Geometry check sheet. Reference: the model listing, model coordinates, mm. A direction names the side the tool comes from. Coordinates: 2 decimals unless noted, no trailing zeros. Loops run counter-clockwise (first coordinate to the right, second up) from the corner with the lowest first, then second, coordinate; pieces in that order, holes last. Notation, with made-up numbers: (65.5, 61.5) -> (108.5, 61.5) arc R20 ccw to (108.5, 77.5) -> close; hole circle Ø8 at (-30, 73.25). An arc over 180 degrees is marked (long way). Answer as a JSON object with one key per item and string values.
from build123d import *

# Parameters (mm, degrees)
SKETCH2_W               = 3.175
SKETCH2_H               = 42.221697185
SKETCH3_W               = 3.175
SKETCH3_H               = 3.175
CUT_EXTRUDE1_DEPTH      = 1.27
CUT_EXTRUDE2_DEPTH      = 41.54574875
CUT_EXTRUDE2_DEPTH_BACK = 41.54574875


with BuildPart() as part:
    # Sketch2 → Revolve1 (revolve)
    with BuildSketch(Plane.XY, mode=Mode.PRIVATE) as revolve1_sk:
        with Locations((22.889936685, 21.110848593)):
            Rectangle(SKETCH2_W, SKETCH2_H)
    revolve(revolve1_sk.sketch.rotate(Axis((0, 38.094197185, 0), (0, -1, 0)), 180), axis=Axis((0, 38.094197185, 0), (0, -1, 0)))

    # Sketch3 → Cut-Extrude1 (cut)
    with BuildSketch(Plane(origin=(0, 42.221697185, 0), x_dir=(1, 0, 0), z_dir=(0, 1, 0))):
        with Locations((0, 24.425903267)):
            Rectangle(SKETCH3_W, SKETCH3_H)
        with Locations((0, -24.425903267)):
            Rectangle(SKETCH3_W, SKETCH3_H)
    cut_extrude1 = extrude(amount=-CUT_EXTRUDE1_DEPTH, mode=Mode.SUBTRACT)

    # Mirror1: Cut-Extrude1 across plane
    add(cut_extrude1.mirror(Plane.ZX.offset(21.110848593)), mode=Mode.SUBTRACT)

    # Sketch4 → Cut-Extrude2 (cut, two sides: drawn at the far end of the back side and taken through both)
    with BuildSketch(Plane(origin=(0, 21.110848593, 0), x_dir=(1, 0, 0), z_dir=(0, 1, 0)).offset(-CUT_EXTRUDE2_DEPTH_BACK)):
        with BuildLine():
            Line((24.472510779, 0.491042627), (23.622, 0))
            Line((23.622, 0), (24.472510779, -0.491042627))
            ThreePointArc((24.472510779, -0.491042627), (24.477436685, 0), (24.472510779, 0.491042627))
        make_face()
        with BuildLine():
            Line((21.26790239, 1.21249192), (23.368, 0))
            Line((23.368, 0), (21.26790239, -1.21249192))
            ThreePointArc((21.26790239, -1.21249192), (21.302436685, 0), (21.26790239, 1.21249192))
        make_face()
    extrude(amount=CUT_EXTRUDE2_DEPTH + CUT_EXTRUDE2_DEPTH_BACK, mode=Mode.SUBTRACT)


solid = part.part
1. Section check C-C, the plane y = 26.5. Record the boundary of the cut face in (x, z).
Evaluation:
{"outline": "(23.62, 0) -> (24.47, 0.49) arc R24.48 ccw (long way) to (24.47, -0.49) -> close; hole (21.27, -1.21) -> (23.37, 0) -> (21.27, 1.21) arc R21.3 ccw (long way) to start"}
2. Mould release check, pull along X, two halves, no side actions. Record for faces 1 (the face through (0, 1, 22.838)), 2 (the face through (0, 42.222, 22)): released by +X, released by -X, zero draft, split by the parting line, or undercut.
Evaluation:
{"face 1": "undercut", "face 2": "zero draft"}
3. Section check D-D, the plane x = 0. Record the boundary of the cut face in (y, z), then the cut area to 3 significant figures.
Evaluation:
{"outline": "(0, -22.84) -> (1.27, -22.84) -> (1.27, -24.48) -> (40.95, -24.48) -> (40.95, -22.84) -> (42.22, -22.84) -> (42.22, -21.3) -> (0, -21.3) -> close; (0, 21.3) -> (42.22, 21.3) -> (42.22, 22.84) -> (40.95, 22.84) -> (40.95, 24.48) -> (1.27, 24.48) -> (1.27, 22.84) -> (0, 22.84) -> close", "area": "260 mm^2"}
4. Section check A-A, the plane x = -19.5. Record the boundary of the cut face in (y, z), then the cut area to 3 significant figures.
Evaluation:
{"outline": "(0, -14.8) -> (42.22, -14.8) -> (42.22, -8.58) -> (0, -8.58) -> close; (0, 8.58) -> (42.22, 8.58) -> (42.22, 14.8) -> (0, 14.8) -> close", "area": "525 mm^2"}
5. Depth check by flat-ended pin: P1, Ø5, axis at x = 19, y = 9.5, coming from the -Z side; P2, Ø1, axis at x = 7, y = 17.5, coming from the +Z side; P3, Ø0.5, axis at x = 0.5, z = 23.5, coming from the -Y side. Enter the tip coordinate at first touch or a pass-through.
Evaluation:
{"P1": "stops at z = -18.08", "P2": "stops at z = 23.6", "P3": "stops at y = 1.27"}
6. Section check B-B, the plane z = -20.5. Record the boundary of the cut face in (x, y), then the cut area to 3 significant figures.
Evaluation:
{"outline": "(-13.38, 0) -> (-5.79, 0) -> (-5.79, 42.22) -> (-13.38, 42.22) -> close; (5.79, 0) -> (13.38, 0) -> (13.38, 42.22) -> (5.79, 42.22) -> close", "area": "640 mm^2"}
7. Tool access check on faces 3 (the face through (1.588, 1, 24)), 4 (the face through (0, 1.27, -24)), 5 (the face through (1.588, 42, 24)), 6 (the face through (1.588, 42, -24)). Record the directions out of +Z, -Z, +X, -X, +Y, -Y that give a thin tool (end or side, any length) a straight path to the whole face; none if there is none.
Evaluation:
{"face 3": "+Z, -Y", "face 4": "-Z, -Y", "face 5": "+Z, +Y", "face 6": "-Z, +Y"}
8. Thickness scan on probe 1 along Z at (x, y) = (-0.5, 13); probe 2 along Z at (x, y) = (11.5, 30.5); probe 3 along X at (y, z) = (24, -9). Record the ranges inside material, lowest first. Write a range as from..to.
Evaluation:
{"probe 1": "z = -24.47..-21.3, 21.3..24.47", "probe 2": "z = -21.61..-17.93, 17.93..21.61", "probe 3": "x = -22.76..-19.31, 19.31..22.76"}
